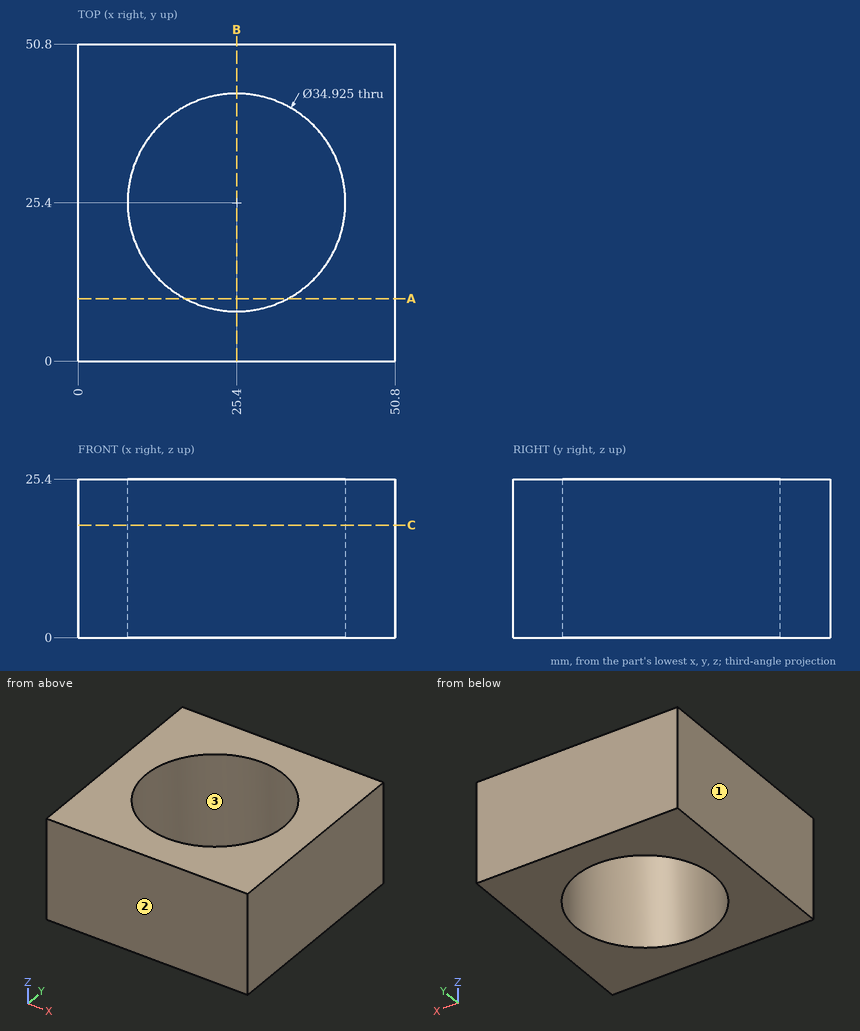
Study the drawing (mm; zero at the part's minimum x, y, z) and answer. Coordinates: 2 decimals unless noted, no trailing zeros. Write each loop counter-clockwise with the first axis right and the second up, starting at its lowest first coordinate (ties: lowest second). Pieces come first, ordered by that corner, then holes.
Q1. Find the intervals of material crossed by line 1 along Y through (x, z) = (25.4, 11.5); line 2 along X through (y, z) = (13, 23.25), in increasing order.
Returned:
line 1: y = 0 to 7.94, 42.86 to 50.8
line 2: x = 0 to 13.1, 37.7 to 50.8
Q2. The mould has two halves that part along X. Classify the marked faces 1, 2 and 3: released by +X, released by -X, zero draft, split by the parting line, or undercut.
Returned:
face 1: released by -X
face 2: zero draft
face 3: undercut
Q3. Section A-A, the plane y = 10 is taken. Write down the section's boundary in (x, z), then the cut area to 3 significant figures.
Returned:
outline: (0, 0) - (17.17, 0) - (17.17, 25.4) - (0, 25.4) - close; (33.63, 0) - (50.8, 0) - (50.8, 25.4) - (33.63, 25.4) - close
area: 872 mm2
Q4. Section B-B, the plane x = 25.4 is taken. Write down the section's boundary in (y, z).
Returned:
outline: (0, 0) - (7.94, 0) - (7.94, 25.4) - (0, 25.4) - close; (42.86, 0) - (50.8, 0) - (50.8, 25.4) - (42.86, 25.4) - close
Q5. Section C-C, the plane z = 18 is taken. Write down the section's boundary in (x, y) (1 decimal), then the cut area to 3 significant figures.
Returned:
outline: (0, 0) - (50.8, 0) - (50.8, 50.8) - (0, 50.8) - close; hole circle Ø34.9 at (25.4, 25.4)
area: 1,620 mm2
